For this review, take the finished solid that the model builds, in its own axes (mm). Round coordinates to 2 decimals unless told otherwise and drop trailing zeros. Write each loop counter-clockwise with the first axis right and the second up, starting at its lowest first coordinate (ties: lowest second). Pieces come first, ordered by that corner, then holes. Notation, with made-up numbers: (83, -28.5) - (141, -28.5) arc R8 cw to (141, -21.5) - close; hole circle Ø7 at (88, -11). An arc over 180 degrees is marked (long way). Answer in a Markdown table with one row per item. Add a question column.
from build123d import *

# Parameters (mm, degrees)
F2_R = 0.35


with BuildPart() as f3:
    # F3: sweep along a path in F0
    with BuildLine(Plane.XY) as f3_path:
        Line((6.55193, 26.69883), (-6.55193, 26.69883))
        ThreePointArc((-6.55193, 26.69883), (-11.8176834888, 24.5176834888), (-13.99883, 19.25193))
        Line((-13.99883, 19.25193), (-13.99883, -19.25193))
        ThreePointArc((-13.99883, -19.25193), (-11.8176834888, -24.5176834888), (-6.55193, -26.69883))
        Line((-6.55193, -26.69883), (6.55193, -26.69883))
        ThreePointArc((6.55193, -26.69883), (11.8176834888, -24.5176834888), (13.99883, -19.25193))
        Line((13.99883, -19.25193), (13.99883, 19.25193))
        ThreePointArc((13.99883, 19.25193), (11.8176834888, 24.5176834888), (6.55193, 26.69883))
    # F2 (on plane+point) → F3 (sweep)
    with BuildSketch(Plane.XZ.offset(19.25193)):
        with Locations((-13.99883, 0)):
            Circle(F2_R)
    sweep(path=f3_path.line)


solid = f3.part
Q1. Add section C-C on x = 6. State the section outline as (y, z) points, then the cut area to 3 significant figures.
Q2. To check wall thickness, follow probe 1 along X at (y, z) = (-19, 0.05); probe 2 along Y at (x, z) = (-4.75, 0.05); probe 3 along Y at (x, z) = (10, 0.1). State the ranges of each line that lie inside material, in increasing order.
Q3. Add section A-A on z = 0. State the section outline as (x, y) points, then the cut area to 3 significant figures.
Q4. Add section B-B on y = 3. State the section outline as (x, z) points.
Answer sheet:
| question | item | result |
|---|---|---|
| 1 | outline | circle Ø0.7 at (-26.7, 0); circle Ø0.7 at (26.7, 0) |
| 1 | area | 0.770 mm² |
| 2 | probe 1 | x = -14.35 to -13.65, 13.65 to 14.35 |
| 2 | probe 2 | y = -27.05 to -26.35, 26.35 to 27.05 |
| 2 | probe 3 | y = -26.23 to -25.47, 25.47 to 26.23 |
| 3 | outline | (-14.35, -19.25) arc R7.8 ccw to (-6.55, -27.05) - (6.55, -27.05) arc R7.8 ccw to (14.35, -19.25) - (14.35, 19.25) arc R7.8 ccw to (6.55, 27.05) - (-6.55, 27.05) arc R7.8 ccw to (-14.35, 19.25) - close; hole (-13.65, -19.25) arc R7.1 ccw to (-6.55, -26.35) - (6.55, -26.35) arc R7.1 ccw to (13.65, -19.25) - (13.65, 19.25) arc R7.1 ccw to (6.55, 26.35) - (-6.55, 26.35) arc R7.1 ccw to (-13.65, 19.25) - close |
| 3 | area | 105 mm² |
| 4 | outline | circle Ø0.7 at (-14, 0); circle Ø0.7 at (14, 0) |
